Check sheet for the modelled part. Datum: model origin and axes. Units: mm. Give positions to 0.01 mm unless a question says otherwise; leave off trailing zeros. Loops run counter-clockwise (first coordinate to the right, second up) from the corner with the lowest first, then second, coordinate; pieces in that order, holes last. Notation, with made-up numbers: (31, 53.5) - (53, 53.5) arc R27 cw to (53, 72.5) - close; hole circle Ø3 at (-5.5, 82.5). An arc over 180 degrees is marked (long way). Answer in a Markdown table with one row per item. Add a question column.
(1) Draft check along Y on faces 1 (the face through (-10, -29, -30.118)), 2 (the face through (-1, 0, 0)), 3 (the face through (-1, -76.2, 0)), 4 (the face through (-3.103, -54.642, 0.422)). Enter one of: released by +Y, released by -Y, zero draft, split by the parting line, or undercut.
(2) Sectioned sample at C-C on z = -10.5. Enter the section's corners in (x, y), then the cut area to 3 significant figures.
(3) Thickness scan on L1, parallel to Y at x = 0, z = 18; L2, parallel to X at y = -50.5, z = 4; L3, parallel to X at y = -36, z = 17. Record the ranges inside material, lowest first.
(4) Sectioned sample at B-B on y = -28.5. Enter the section's corners in (x, z), then the cut area to 3 significant figures.
(5) Go/stop test with a flat-tipped pin: P1, Ø8, axis at x = -4.5, z = 19.5, coming from the +Y side. Record where the tip stops, or that it passes through.
(6) Sectioned sample at A-A on x = 0. Enter the section's corners in (y, z).
from build123d import *

# Parameters (mm, degrees)
F0_W     = 81.543564
F0_H     = 60.235682
F1_DEPTH = 76.2
F2_R     = 14.31333
F3_DEPTH = 63.5


with BuildPart() as f1:
    # F0 (on Front) → F1 (new body)
    with BuildSketch(Plane.XZ):
        Rectangle(F0_W, F0_H)
    extrude(amount=F1_DEPTH)

    # F2 (on face) → F3 (cut, symmetric)
    with BuildSketch(Plane.XY.offset(30.117841)):
        with Locations((0, -40.668592)):
            Circle(F2_R)
    extrude(amount=F3_DEPTH, both=True, mode=Mode.SUBTRACT)


solid = f1.part
Reply:
| question | item | result |
|---|---|---|
| 1 | face 1 | zero draft |
| 1 | face 2 | released by +Y |
| 1 | face 3 | released by -Y |
| 1 | face 4 | undercut |
| 2 | outline | (-40.77, -76.2) - (40.77, -76.2) - (40.77, 0) - (-40.77, 0) - close; hole circle Ø28.63 at (0, -40.67) |
| 2 | area | 5,570 mm^2 |
| 3 | L1 | -76.2 to -54.98, -26.36 to 0 |
| 3 | L2 | -40.77 to -10.4, 10.4 to 40.77 |
| 3 | L3 | -40.77 to -13.53, 13.53 to 40.77 |
| 4 | outline | (-40.77, -30.12) - (-7.54, -30.12) - (-7.54, 30.12) - (-40.77, 30.12) - close; (7.54, -30.12) - (40.77, -30.12) - (40.77, 30.12) - (7.54, 30.12) - close |
| 4 | area | 4,000 mm^2 |
| 5 | P1 | y = 0 |
| 6 | outline | (-76.2, -30.12) - (-54.98, -30.12) - (-54.98, 30.12) - (-76.2, 30.12) - close; (-26.36, -30.12) - (0, -30.12) - (0, 30.12) - (-26.36, 30.12) - close |
